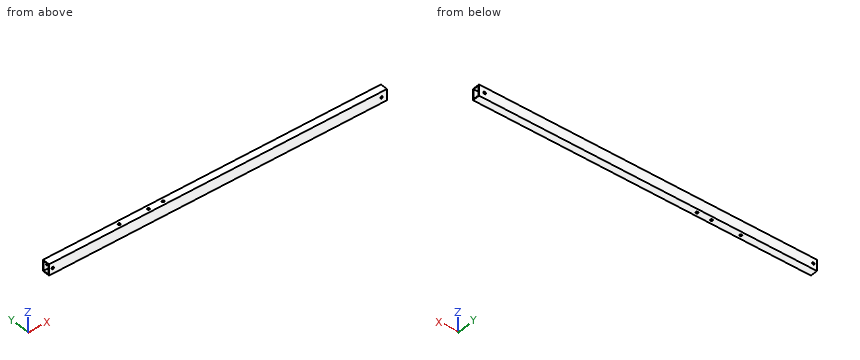
from build123d import *

# Parameters (mm, degrees)
SKETCH_1_W          = 220
SKETCH_1_H          = 10
SKETCH_1_R          = 1.6
EXTRUDE_1_DEPTH     = 15
SKETCH_2_W          = 13
SKETCH_2_H          = 8
CUT_EXTRUDE_1_DEPTH = 2000
SKETCH_3_R          = 1.6
CUT_EXTRUDE_2_DEPTH = 1000
SKETCH_7_W          = 242
SKETCH_7_H          = 15
SKETCH_7_R          = 1.6
EXTRUDE_3_DEPTH     = 10
SKETCH_8_W          = 13
SKETCH_8_H          = 8
CUT_EXTRUDE_4_DEPTH = 1000


with BuildPart() as part:
    # ｽｹｯﾁ1 → ﾎﾞｽ - 押し出し1 (new body)
    with BuildSketch(Plane.XY):
        with Locations((-610, 0)):
            Rectangle(SKETCH_1_W, SKETCH_1_H)
        with Locations((-620, 0)):
            Circle(SKETCH_1_R, mode=Mode.SUBTRACT)
        with Locations((-580, 0)):
            Circle(SKETCH_1_R, mode=Mode.SUBTRACT)
        with Locations((-560, 0)):
            Circle(SKETCH_1_R, mode=Mode.SUBTRACT)
    extrude(amount=EXTRUDE_1_DEPTH)

    # ｽｹｯﾁ2 → ｶｯﾄ - 押し出し1 (cut)
    with BuildSketch(Plane(origin=(-500, 0, 0), x_dir=(0, 0, -1), z_dir=(1, 0, 0))):
        with Locations((-7.5, 0)):
            Rectangle(SKETCH_2_W, SKETCH_2_H)
    extrude(amount=-CUT_EXTRUDE_1_DEPTH, mode=Mode.SUBTRACT)

    # ｽｹｯﾁ3 → ｶｯﾄ - 押し出し2 (cut)
    with BuildSketch(Plane(origin=(0, -5, 0), x_dir=(-1, 0, 0), z_dir=(0, -1, 0))):
        with Locations(Location((715, -7.5, 0), (0, 0, 180))):
            Circle(SKETCH_3_R)
    extrude(amount=-CUT_EXTRUDE_2_DEPTH, mode=Mode.SUBTRACT)

    # ｽｹｯﾁ7 → ﾎﾞｽ - 押し出し3 (add)
    with BuildSketch(Plane.XZ.offset(5)):
        with Locations((-379, 7.5)):
            Rectangle(SKETCH_7_W, SKETCH_7_H)
        with Locations((-265.5, 7.5)):
            Circle(SKETCH_7_R, mode=Mode.SUBTRACT)
    extrude(amount=-EXTRUDE_3_DEPTH)

    # ｽｹｯﾁ8 → ｶｯﾄ - 押し出し4 (cut)
    with BuildSketch(Plane.ZY.offset(720)):
        with Locations((7.5, 0)):
            Rectangle(SKETCH_8_W, SKETCH_8_H)
    extrude(amount=-CUT_EXTRUDE_4_DEPTH, mode=Mode.SUBTRACT)


solid = part.part
The listing builds one solid part. Answer for the finished solid, in the listing's coordinates (mm). Coordinates: 2 decimals unless noted, no trailing zeros. Write each loop counter-clockwise with the first axis right and the second up, starting at its lowest first coordinate (ties: lowest second). Pieces come first, ordered by that corner, then holes. Notation, with made-up numbers: M 75,-15.75 L 111,-15.75 A24 ccw 111,-3.75 Z; hole C 9,18 d6. An arc over 180 degrees is marked long. Put each result on its own line as item: value. Start each with the question number.
1. Consider line 1 (X direction, y = 0, z = 14.65); line 2 (Z direction, x = -450.5, y = -2); line 3 (Y direction, x = -548.5, z = 3.25). Determine where each line is inside the solid, lowest interval first. Write a range as from..to.
2. A cutting plane is placed at B-B on x = -643. Write down the section's boundary in (y, z).
3. A cutting plane is placed at A-A on z = 3.5. Write down the section's boundary in (x, y).
Resolved:
1. line 1: x = -720..-621.6, -618.4..-581.6, -578.4..-561.6, -558.4..-258
1. line 2: z = 0..1, 14..15
1. line 3: y = -5..-4, 4..5
2. outline: M -5,0 L 5,0 L 5,15 L -5,15 Z; hole M -4,1 L 4,1 L 4,14 L -4,14 Z
3. outline: M -720,-5 L -258,-5 L -258,-4 L -720,-4 Z; M -720,4 L -258,4 L -258,5 L -720,5 Z
